Work out the finished part from the listing and answer in its coordinate system (mm). Face numbers are marked on the shaded views. A direction names the side the tool comes from. Coordinates: 2 decimals unless noted, no trailing zeros. Write each loop counter-clockwise with the first axis right and the second up, starting at its lowest first coordinate (ties: lowest second). Pieces come first, ordered by that corner, then holes. Notation, with made-up numbers: M 69.25,68.5 L 98.25,68.5 A34 cw 98.25,98.5 Z; hole C 22,-7 d8. An arc over 180 degrees is marked long. Answer as CSV lines item,"result". Start each with the question number.
(1) Flat-ended cylindrical pins translate along their axes: P1, Ø6, axis at x = -50.5, z = 52, coming from the +Y side (3 decimals); P2, Ø8, axis at y = -202.5, z = 50, coming from the +X side; P3, Ø2, axis at x = -76, z = 46.5, coming from the +Y side; P4, Ø7.5, axis at x = 92.62, y = -19.5, coming from the +Z side. Find the tip coordinate at first contact, or state that the pin passes through.
(2) Find the intervals of material crossed by L1, parallel to X at y = -188.5, z = 44.5; L2, parallel to Y at x = 31.5, z = 9; L3, parallel to Y at x = 129, z = 39.5, in increasing order. Write a range as [from, to].
(3) A cutting plane is placed at B-B on y = -185. Give the vertices of the cut face in (x, z), then the cut area to 3 significant figures.
(4) A cutting plane is placed at C-C on z = 59.5. Give the vertices of the cut face in (x, y).
(5) A cutting plane is placed at D-D on y = -152. Give the vertices of the cut face in (x, z), then the cut area to 3 significant figures.
(6) The mould has two halves that part along Y. Classify the marked faces 3, 4, 5 and 6: released by +Y, released by -Y, zero draft, split by the parting line, or undercut.
(7) A cutting plane is placed at A-A on x = 29. Give the vertices of the cut face in (y, z), then the cut area to 3 significant figures.
(8) For the marked faces 1 and 2, determine the directions among +Z, -Z, +X, -X, +Y, -Y from which every point of the face is accessible in a straight line to the end or side of a thin tool.
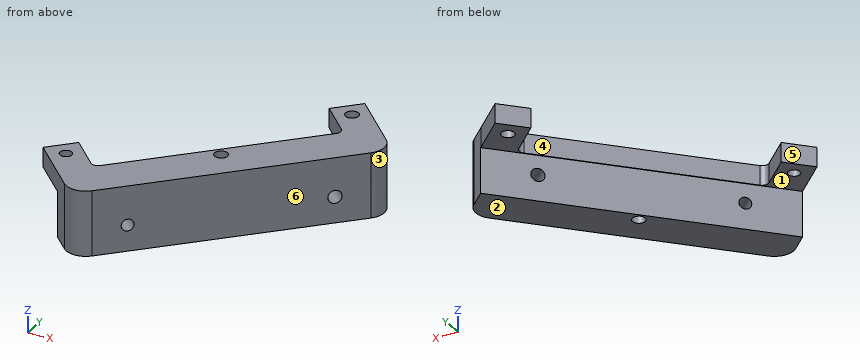
from build123d import *

# Parameters (mm, degrees)
SKETCH1_R                         = 6.35
BASE_EXTRUDE_DEPTH                = 63.5
SKETCH2_W                         = 45.301656397
SKETCH2_H                         = 44.45
CUT_EXTRUDE1_DEPTH                = 324.049195456
F_1_2_20_TAPPED_HOLE4_D           = 11.50874
F_1_2_20_TAPPED_HOLE3_D           = 11.50874
F_1_2_20_TAPPED_HOLE3_CBORE_D     = 12.7
F_1_2_20_TAPPED_HOLE3_CBORE_DEPTH = 25.4
F_1_2_20_TAPPED_HOLE1_D           = 12.7
F_1_2_20_TAPPED_HOLE2_D           = 11.50874


with BuildPart() as part:
    # Sketch1 → Base-Extrude (new body)
    with BuildSketch(Plane.XY):
        with BuildLine():
            Line((-87.034046036, -176.655263526), (-109.476853925, -199.11373351))
            Line((-109.476853925, -199.11373351), (-62.270703318, -246.286963476))
            ThreePointArc((-62.270703318, -246.286963476), (-48.800588675, -251.86188097), (-35.333068284, -246.280699366))
            Line((-35.333068284, -246.280699366), (139.761564896, -71.145344736))
            ThreePointArc((139.761564896, -71.145344736), (145.339614596, -57.676526855), (139.761564896, -44.207708974))
            Line((139.761564896, -44.207708974), (124.048977285, -28.491467114))
            Line((124.048977285, -28.491467114), (92.616039983, 2.948780491))
            Line((92.616039983, 2.948780491), (70.168405011, -19.504866145))
            Line((70.168405011, -19.504866145), (97.107164721, -46.449890955))
            ThreePointArc((97.107164721, -46.449890955), (98.966514621, -50.939440985), (97.107243808, -55.429023769))
            Line((97.107243808, -55.429023769), (-51.056538279, -203.63248535))
            ThreePointArc((-51.056538279, -203.63248535), (-55.545734899, -205.492958311), (-60.035829043, -203.634652493))
            Line((-60.035829043, -203.634652493), (-87.034046036, -176.655263526))
        make_face()
        with Locations((29.591473015, -136.091254995)):
            Circle(SKETCH1_R, mode=Mode.SUBTRACT)
    extrude(amount=BASE_EXTRUDE_DEPTH)

    # Sketch2 → Cut-Extrude1 (cut, through all)
    with BuildSketch(Plane(origin=(-154.257082678, -154.364733609, 0), x_dir=(0.707353385, -0.706860091, 0), z_dir=(-0.706860091, -0.707353385, 0))):
        with Locations((85.957556745, 22.225)):
            Rectangle(SKETCH2_W, SKETCH2_H)
    extrude(amount=-CUT_EXTRUDE1_DEPTH, mode=Mode.SUBTRACT)

    # 1/2-20 Tapped Hole4 (through all)
    with Locations(Plane.XY.offset(63.5)):
        with Locations((-87.026214989, -199.105902462)):
            Hole(F_1_2_20_TAPPED_HOLE4_D / 2)

    # 1/2-20 Tapped Hole3 (through all)
    with Locations(Plane.XY.offset(63.5)):
        with Locations((92.616237749, -19.504668428)):
            CounterBoreHole(F_1_2_20_TAPPED_HOLE3_D / 2, F_1_2_20_TAPPED_HOLE3_CBORE_D / 2, F_1_2_20_TAPPED_HOLE3_CBORE_DEPTH)

    # 1/2-20 Tapped Hole1 (through all)
    with Locations(Plane(origin=(105.469704015, -105.445180815, 0), x_dir=(0, 0, -1), z_dir=(0.707188992, -0.707024561, 0))):
        with Locations((-25.4, 16.751653867)):
            Hole(F_1_2_20_TAPPED_HOLE1_D / 2)

    # 1/2-20 Tapped Hole2 (through all)
    with Locations(Plane(origin=(105.469704015, -105.445180815, 0), x_dir=(0, 0, -1), z_dir=(0.707188992, -0.707024561, 0))):
        with Locations((-25.4, -167.398346133)):
            Hole(F_1_2_20_TAPPED_HOLE2_D / 2)


solid = part.part
Here are the results:
1,P1,"stops at y = -200.075"
1,P2,"stops at x = 12.44"
1,P3,"stops at y = -186.68"
1,P4,"passes through"
2,L1,"x = [-98.87, -75.18], [-35.93, 22.43]"
2,L2,"y = [-179.43, -142.15], [-130.03, -122.13]"
2,L3,"y = [-81.91, -33.44]"
3,outline,"M -95.37,44.45 L -78.68,44.45 L -78.68,63.5 L -95.37,63.5 Z; M -32.43,44.45 L -31.33,44.45 L -31.33,0 L 25.93,0 L 25.93,63.5 L -32.43,63.5 Z"
3,area,"3,980 mm^2"
4,outline,"M -109.48,-199.11 L -62.27,-246.29 A19.05 ccw -35.33,-246.28 L 139.76,-71.15 A19.05 ccw 139.76,-44.21 L 92.62,2.95 L 70.17,-19.5 L 97.11,-46.45 A6.35 cw 97.11,-55.43 L -51.06,-203.63 A6.35 cw -60.04,-203.63 L -87.03,-176.66 Z; hole C -87.03,-199.11 d11.51; hole C 29.59,-136.09 d12.7; hole C 92.62,-19.5 d12.7"
5,outline,"M 0.56,44.45 L 1.65,44.45 L 1.65,0 L 58.93,0 L 58.93,63.5 L 0.56,63.5 Z"
5,area,"3,660 mm^2"
6,face 3,"split by the parting line"
6,face 4,"undercut"
6,face 5,"released by +Y"
6,face 6,"released by -Y"
7,outline,"M -181.93,0 L -142.41,0 L -142.41,63.5 L -181.93,63.5 Z; M -129.77,0 L -124.63,0 L -124.63,44.45 L -123.55,44.45 L -123.55,63.5 L -129.77,63.5 Z"
7,area,"2,860 mm^2"
8,face 1,"-Z, -X, +Y"
8,face 2,"-Z, +X, -X, +Y, -Y"
